from build123d import *

# Parameters (mm, degrees)
F1_DEPTH  = 80
F3_DEPTH  = 2
F5_DEPTH  = 2
F7_DEPTH  = 2
F9_DEPTH  = 2
F10_R     = 2.5
F11_DEPTH = 1
F13_DEPTH = 2
F14_W     = 9
F14_H     = 5
F15_DEPTH = 3
F16_R     = 2
F17_DEPTH = 2


with BuildPart() as f1:
    # F0 (on Right) → F1 (new body)
    with BuildSketch(Plane.YZ):
        with BuildLine():
            Line((56.9827339551, -40.4682084375), (56.9827339551, 39.5317915625))
            Line((56.9827339551, 39.5317915625), (-13.0172660449, 39.5317915625))
            Line((-13.0172660449, 39.5317915625), (-23.0172660449, -10.4682084375))
            Line((-23.0172660449, -10.4682084375), (-63.0172660449, -10.4682084375))
            Line((-63.0172660449, -10.4682084375), (-63.0172660449, -40.4682084375))
            Line((-63.0172660449, -40.4682084375), (-41.4112906903, -40.4682084375))
            ThreePointArc((-41.4112906903, -40.4682084375), (-28.9112906903, -27.9682084375), (-16.4112906903, -40.4682084375))
            Line((-16.4112906903, -40.4682084375), (18.5887116939, -40.4682084375))
            ThreePointArc((18.5887116939, -40.4682084375), (31.0887116939, -27.9682084375), (43.5887116939, -40.4682084375))
            Line((43.5887116939, -40.4682084375), (56.9827339551, -40.4682084375))
        make_face()
        with BuildLine():
            Line((-41.4112906903, -40.4682084375), (-16.4112906903, -40.4682084375))
            ThreePointArc((-16.4112906903, -40.4682084375), (-28.9112906903, -27.9682084375), (-41.4112906903, -40.4682084375))
        make_face()
        with BuildLine():
            ThreePointArc((-41.4112906903, -40.4682084375), (-28.9112906903, -52.9682084375), (-16.4112906903, -40.4682084375))
            Line((-16.4112906903, -40.4682084375), (-41.4112906903, -40.4682084375))
        make_face()
        with BuildLine():
            ThreePointArc((18.5887116939, -40.4682084375), (31.0887116939, -52.9682084375), (43.5887116939, -40.4682084375))
            Line((43.5887116939, -40.4682084375), (18.5887116939, -40.4682084375))
        make_face()
        with BuildLine():
            Line((18.5887116939, -40.4682084375), (43.5887116939, -40.4682084375))
            ThreePointArc((43.5887116939, -40.4682084375), (31.0887116939, -27.9682084375), (18.5887116939, -40.4682084375))
        make_face()
    extrude(amount=F1_DEPTH)

    # F2 (on face) → F3 (cut)
    with BuildSketch(Plane.YZ.offset(80)):
        Polygon((49.9866685293, 31.5270468074), (0, 30.3725038928), (-10.0133314707, -12.4729531926), (49.9866685293, -12.4729531926), align=None)
    extrude(amount=-F3_DEPTH, mode=Mode.SUBTRACT)

    # F4 (on face) → F5 (cut)
    with BuildSketch(Plane(origin=(0, 0, 0), x_dir=(0, -1, 0), z_dir=(-1, 0, 0))):
        Polygon((10.0133314707, -9.3607458684), (0, 33.484711217), (-49.9866685293, 34.6392541316), (-49.9866685293, -9.3607458684), align=None)
    extrude(amount=-F5_DEPTH, mode=Mode.SUBTRACT)

    # F6 (on face) → F7 (cut)
    with BuildSketch(Plane(origin=(0, -20.1188695744, 4.0237739149), x_dir=(1, 0, 0), z_dir=(0, -0.9805806757, 0.1961161351))):
        with BuildLine():
            ThreePointArc((12.5413901359, 28.6179297172), (9.00585623, 27.1534636231), (7.5413901359, 23.6179297172))
            Line((7.5413901359, 23.6179297172), (7.5413901359, -11.3820702828))
            Line((7.5413901359, -11.3820702828), (72.5413901359, -11.3820702828))
            Line((72.5413901359, -11.3820702828), (72.5413901359, 23.6179297172))
            ThreePointArc((72.5413901359, 23.6179297172), (71.0769240418, 27.1534636231), (67.5413901359, 28.6179297172))
            Line((67.5413901359, 28.6179297172), (12.5413901359, 28.6179297172))
        make_face()
    extrude(amount=-F7_DEPTH, mode=Mode.SUBTRACT)

    # F8 (on face) → F9 (join)
    with BuildSketch(Plane.XZ.offset(63.0172660449)):
        with BuildLine():
            ThreePointArc((16.8799156292, -28.4473337126), (16.5870224104, -27.7402269314), (15.8799156292, -27.4473337126))
            Line((15.8799156292, -27.4473337126), (8.8799156292, -27.4473337126))
            ThreePointArc((8.8799156292, -27.4473337126), (8.172808848, -27.7402269314), (7.8799156292, -28.4473337126))
            Line((7.8799156292, -28.4473337126), (7.8799156292, -31.4473337126))
            ThreePointArc((7.8799156292, -31.4473337126), (8.172808848, -32.1544404937), (8.8799156292, -32.4473337126))
            Line((8.8799156292, -32.4473337126), (15.8799156292, -32.4473337126))
            ThreePointArc((15.8799156292, -32.4473337126), (16.5870224104, -32.1544404937), (16.8799156292, -31.4473337126))
            Line((16.8799156292, -31.4473337126), (16.8799156292, -28.4473337126))
        make_face()
        with BuildLine():
            ThreePointArc((68.5099807539, -28.4473337126), (68.2170875351, -27.7402269314), (67.5099807539, -27.4473337126))
            Line((67.5099807539, -27.4473337126), (60.5099807539, -27.4473337126))
            ThreePointArc((60.5099807539, -27.4473337126), (59.8028739727, -27.7402269314), (59.5099807539, -28.4473337126))
            Line((59.5099807539, -28.4473337126), (59.5099807539, -31.4473337126))
            ThreePointArc((59.5099807539, -31.4473337126), (59.8028739727, -32.1544404937), (60.5099807539, -32.4473337126))
            Line((60.5099807539, -32.4473337126), (67.5099807539, -32.4473337126))
            ThreePointArc((67.5099807539, -32.4473337126), (68.2170875351, -32.1544404937), (68.5099807539, -31.4473337126))
            Line((68.5099807539, -31.4473337126), (68.5099807539, -28.4473337126))
        make_face()
    extrude(amount=F9_DEPTH)

    # F10 (on face) → F11 (join)
    with BuildSketch(Plane.XZ.offset(63.0172660449)):
        with Locations((21.8240363776, -30.4359253496)):
            Circle(F10_R)
        with Locations((53.2039631238, -30.4221354475)):
            Circle(F10_R)
    extrude(amount=F11_DEPTH)

    # F12 (on face) → F13 (cut)
    with BuildSketch(Plane(origin=(0, 56.9827339551, 0), x_dir=(-1, 0, 0), z_dir=(0, 1, 0))):
        with BuildLine():
            Line((-11.3534486648, 31.5445680549), (-71.3534486648, 31.5445680549))
            ThreePointArc((-71.3534486648, 31.5445680549), (-73.4747690083, 30.6658883985), (-74.3534486648, 28.5445680549))
            Line((-74.3534486648, 28.5445680549), (-74.3534486648, -3.4554319451))
            Line((-74.3534486648, -3.4554319451), (-8.3534486648, -3.4554319451))
            Line((-8.3534486648, -3.4554319451), (-8.3534486648, 28.5445680549))
            ThreePointArc((-8.3534486648, 28.5445680549), (-9.2321283212, 30.6658883985), (-11.3534486648, 31.5445680549))
        make_face()
    extrude(amount=-F13_DEPTH, mode=Mode.SUBTRACT)

    # F14 (on face) → F15 (join)
    with BuildSketch(Plane(origin=(0, 56.9827339551, 0), x_dir=(-1, 0, 0), z_dir=(0, 1, 0))):
        with Locations((-66.6173999912, -29.532836911)):
            Rectangle(F14_W, F14_H)
        with Locations((-15.7938591157, -29.8857766254)):
            Rectangle(F14_W, F14_H)
    extrude(amount=F15_DEPTH)

    # F16 (on face) → F17 (join)
    with BuildSketch(Plane(origin=(0, 56.9827339551, 0), x_dir=(-1, 0, 0), z_dir=(0, 1, 0))):
        with Locations((-24.1537547966, -30.3156095468)):
            Circle(F16_R)
        with Locations((-58.2354065123, -29.9409476741)):
            Circle(F16_R)
    extrude(amount=F17_DEPTH)


solid = f1.part
Work out the finished part from the listing and answer in its coordinate system (mm). A direction names the side the tool comes from. Coordinates: 2 decimals unless noted, no trailing zeros. Write each loop counter-clockwise with the first axis right and the second up, starting at its lowest first coordinate (ties: lowest second). Pieces come first, ordered by that corner, then holes. Notation, with made-up numbers: M -11,12.5 L 23,12.5 A23 cw 23,24.5 Z; hole C 39,51 d3. An arc over 180 degrees is marked long. Use one line per item in the form item = value. Start each with the question number.
1. The part is cut by section C-C (y = 41). Give the vertices of the cut face in (x, z).
2. The mould has two halves that part along X. Classify faces 1 (the face through (78, 20, 10)), 2 (the face through (67, 59.983, -29)), 3 (the face through (19.84, -63.51, -31.96)): released by +X, released by -X, zero draft, split by the parting line, or undercut.
3. The part is cut by section A-A (x = 64). Give the vertices of the cut face in (y, z).
4. Straight lines are drawn through the part: probe 1 along Y at (x, z) = (73, -33); probe 2 along Z at (x, y) = (40, -8.5); probe 3 along Z at (x, y) = (8.5, -53.5). For each, find the intervals that lie inside material, in ascending order. Write a range as from..to.
5. The part is cut by section B-B (z = 22). Give the vertices of the cut face in (x, y), plus the area to 3 significant figures.
6. A tool of negligible diameter and unlimited length cuts with its end or side. For faces 4 (the face through (51.22, -63.51, -31.94)), 5 (the face through (16, 58, -32.386)), 6 (the face through (20.294, 58, -30)), 7 (the face through (39, -43, -10.468)), from which of +Z, -Z, +X, -X, +Y, -Y can it reach the whole face along a straight path? Write none if from no direction.
7. The part is cut by section D-D (x = 48). Give the vertices of the cut face in (y, z).
8. Each of these flat-tipped pins is pushed along its axis until it touches: P1, Ø1.5, axis at x = 13, y = -32.5, coming from the -Z side; P2, Ø1, axis at y = -64.5, z = -30, coming from the +X side; P3, Ø8, axis at x = 23, z = 9.5, coming from the -Y side. Where does it stop, or does it pass through?
Evaluation:
q1.outline = M 0,-48.09 L 80,-48.09 L 80,-12.47 L 78,-12.47 L 78,31.32 L 80,31.32 L 80,39.53 L 0,39.53 L 0,34.43 L 2,34.43 L 2,-9.36 L 0,-9.36 Z
q2.face_1 = released by +X
q2.face_2 = zero draft
q2.face_3 = undercut
q3.outline = M -65.02,-32.45 L -63.02,-32.45 L -63.02,-40.47 L -41.41,-40.47 A12.5 ccw -16.41,-40.47 L 18.59,-40.47 A12.5 ccw 43.59,-40.47 L 56.98,-40.47 L 56.98,-32.03 L 59.98,-32.03 L 59.98,-27.03 L 56.98,-27.03 L 56.98,-3.46 L 54.98,-3.46 L 54.98,31.54 L 56.98,31.54 L 56.98,39.53 L -13.02,39.53 L -14.51,32.09 L -12.55,31.69 L -20.39,-7.53 L -22.35,-7.14 L -23.02,-10.47 L -63.02,-10.47 L -63.02,-27.45 L -65.02,-27.45 Z
q4.probe_1 = -63.02..56.98
q4.probe_2 = -40.47..39.53
q4.probe_3 = -40.47..-10.47
q5.outline = M 0,-16.52 L 7.54,-16.52 L 7.54,-14.48 L 72.54,-14.48 L 72.54,-16.52 L 80,-16.52 L 80,-1.96 L 78,-1.96 L 78,49.99 L 80,49.99 L 80,56.98 L 74.35,56.98 L 74.35,54.98 L 8.35,54.98 L 8.35,56.98 L 0,56.98 L 0,49.99 L 2,49.99 L 2,-2.68 L 0,-2.68 Z
q5.area = 5,410 mm^2
q6.face_4 = -Y
q6.face_5 = -Z, +X, -X, +Y
q6.face_6 = +Z, -Z, +Y
q6.face_7 = +Z, +X, -X, -Y
q7.outline = M -63.02,-40.47 L -41.41,-40.47 A12.5 ccw -16.41,-40.47 L 18.59,-40.47 A12.5 ccw 43.59,-40.47 L 56.98,-40.47 L 56.98,-3.46 L 54.98,-3.46 L 54.98,31.54 L 56.98,31.54 L 56.98,39.53 L -13.02,39.53 L -14.51,32.09 L -12.55,31.69 L -20.39,-7.53 L -22.35,-7.14 L -23.02,-10.47 L -63.02,-10.47 Z
q8.P1 = -52.64
q8.P2 = 68.51
q8.P3 = -17.78
